Autodesk Fusion 360 part; units mm, degrees
sketch "Sketch1" plane through (0, 0, 0) normal (0, 1, 0) x (1, 0, 0)
  line L0 (-67.5, -70) -> (67.5, -70)
  line L1 (70, -67.5) -> (70, 67.5)
  line L2 (67.5, 70) -> (-67.5, 70)
  line L3 (-70, 67.5) -> (-70, -67.5)
  line L4 (-70, -70) -> (70, 70) construction
  line L5 (70, -70) -> (-70, 70) construction
  arc A0 (-67.5, 70) -> (-70, 67.5) centre (-67.5, 67.5) ccw
  arc A1 (70, 67.5) -> (67.5, 70) centre (67.5, 67.5) ccw
  arc A2 (67.5, -70) -> (70, -67.5) centre (67.5, -67.5) ccw
  arc A3 (-70, -67.5) -> (-67.5, -70) centre (-67.5, -67.5) ccw
  dimension "d1" = 140
  dimension "d2" = 140
  dimension "d25" = 2.5
  dimension "d26" = 2.5
  dimension "d27" = 2.5
  dimension "d28" = 2.5
extrude "Extrude1" add sketch "Sketch1" along normal blind 3
sketch "Sketch11" plane through (0, 0, 0) normal (0, -1, 0) x (1, 0, 0)
  arc A0 (-67.5, 70) -> (-70, 67.5) centre (-67.5, 67.5) ccw
  line L0 (-70, 67.5) -> (-70, -67.5)
  arc A1 (-70, -67.5) -> (-67.5, -70) centre (-67.5, -67.5) ccw
  line L1 (-67.5, -70) -> (67.5, -70)
  arc A2 (67.5, -70) -> (70, -67.5) centre (67.5, -67.5) ccw
  line L2 (70, -67.5) -> (70, 67.5)
  arc A3 (70, 67.5) -> (67.5, 70) centre (67.5, 67.5) ccw
  line L3 (67.5, 70) -> (-67.5, 70)
  line L4 (37.5, 38.65) -> (37.5, 51.35)
  line L5 (-37.5, 51.35) -> (-37.5, 38.65)
  line L6 (-51.35, -37.5) -> (-38.65, -37.5)
  line L7 (-38.65, 37.5) -> (-51.35, 37.5)
  line L8 (37.5, -51.35) -> (37.5, -38.65)
  line L9 (-37.5, -38.65) -> (-37.5, -51.35)
  line L10 (38.65, -37.5) -> (51.35, -37.5)
  line L11 (51.35, 37.5) -> (38.65, 37.5)
  circle A4 centre (-22, -45) radius 2.1
  circle A5 centre (-32, -45) radius 2.1
  circle A6 centre (22, -45) radius 2.1
  circle A7 centre (32, -45) radius 2.1
  circle A8 centre (-45, -22) radius 2.1
  circle A9 centre (-45, -32) radius 2.1
  circle A10 centre (-45, 22) radius 2.1
  circle A11 centre (-45, 32) radius 2.1
  circle A12 centre (-32, 45) radius 2.1
  circle A13 centre (-22, 45) radius 2.1
  circle A14 centre (22, 45) radius 2.1
  circle A15 centre (32, 45) radius 2.1
  circle A16 centre (45, 22) radius 2.1
  circle A17 centre (45, 32) radius 2.1
  circle A18 centre (45, -22) radius 2.1
  circle A19 centre (45, -32) radius 2.1
  line L12 (-51.35, 37.5) -> (-38.65, 37.5)
  line L13 (-38.65, 37.5) -> (-38.65, 16.5)
  line L14 (-38.65, 16.5) -> (-51.35, 16.5)
  line L15 (-51.35, 16.5) -> (-51.35, 37.5)
  line L16 (-51.35, -37.5) -> (-38.65, -37.5)
  line L17 (-38.65, -37.5) -> (-38.65, -16.5)
  line L18 (-38.65, -16.5) -> (-51.35, -16.5)
  line L19 (-51.35, -16.5) -> (-51.35, -37.5)
  line L20 (-37.5, -51.35) -> (-16.5, -51.35)
  line L21 (-16.5, -51.35) -> (-16.5, -38.65)
  line L22 (-16.5, -38.65) -> (-37.5, -38.65)
  line L23 (-37.5, -38.65) -> (-37.5, -51.35)
  line L24 (37.5, -38.65) -> (16.5, -38.65)
  line L25 (16.5, -38.65) -> (16.5, -51.35)
  line L26 (16.5, -51.35) -> (37.5, -51.35)
  line L27 (37.5, -51.35) -> (37.5, -38.65)
  line L28 (38.65, -37.5) -> (51.35, -37.5)
  line L29 (51.35, -37.5) -> (51.35, -16.5)
  line L30 (51.35, -16.5) -> (38.65, -16.5)
  line L31 (38.65, -16.5) -> (38.65, -37.5)
  line L32 (51.35, 37.5) -> (38.65, 37.5)
  line L33 (38.65, 37.5) -> (38.65, 16.5)
  line L34 (38.65, 16.5) -> (51.35, 16.5)
  line L35 (51.35, 16.5) -> (51.35, 37.5)
  line L36 (37.5, 38.65) -> (16.5, 38.65)
  line L37 (16.5, 38.65) -> (16.5, 51.35)
  line L38 (16.5, 51.35) -> (37.5, 51.35)
  line L39 (37.5, 51.35) -> (37.5, 38.65)
  line L40 (-37.5, 38.65) -> (-16.5, 38.65)
  line L41 (-16.5, 38.65) -> (-16.5, 51.35)
  line L42 (-16.5, 51.35) -> (-37.5, 51.35)
  line L43 (-37.5, 51.35) -> (-37.5, 38.65)
  point P0 (0, 45)
  point P1 (-45, 0)
  point P2 (45, 0)
  dimension "d68" = 12.7
  dimension "d73" = 12.7
  dimension "d77" = 4.2
  dimension "d79" = 4.2
  dimension "d81" = 4.2
  dimension "d83" = 4.2
  dimension "d85" = 4.2
  dimension "d87" = 4.2
  dimension "d89" = 4.2
  dimension "d91" = 4.2
  dimension "d93" = 4.2
  dimension "d95" = 4.2
  dimension "d97" = 4.2
  dimension "d99" = 4.2
  dimension "d101" = 4.2
  dimension "d103" = 4.2
  dimension "d105" = 4.2
  dimension "d107" = 4.2
  dimension "d111" = 21
  dimension "d112" = 12.7
  dimension "d113" = 21
  dimension "d114" = 21
  dimension "d115" = 21
  dimension "d116" = 21
  dimension "d117" = 21
  dimension "d118" = 21
  dimension "d119" = 21
  dimension "d120" = 12.7
extrude "Extrude9" add sketch "Sketch11" along normal blind 5 contours L5 L40 L41 L42 L43 | L6 L16 L17 L18 L19 | L8 L24 L25 L26 L27 | L11 L32 L33 L34 L35
sketch "Sketch14" plane through (0, 0, 0) normal (0, -1, 0) x (-1, 0, 0)
  line L0 (51.35, 16.5) -> (38.65, 16.5)
  line L1 (38.65, 16.5) -> (38.65, 37.5)
  line L2 (38.65, 37.5) -> (51.35, 37.5)
  line L3 (51.35, 37.5) -> (51.35, 16.5)
  line L4 (37.5, -51.35) -> (16.5, -51.35)
  line L5 (16.5, -51.35) -> (16.5, -38.65)
  line L6 (16.5, -38.65) -> (37.5, -38.65)
  line L7 (37.5, -38.65) -> (37.5, -51.35)
  line L8 (-37.5, 51.35) -> (-16.5, 51.35)
  line L9 (-16.5, 51.35) -> (-16.5, 38.65)
  line L10 (-16.5, 38.65) -> (-37.5, 38.65)
  line L11 (-37.5, 38.65) -> (-37.5, 51.35)
  line L12 (-51.35, -16.5) -> (-38.65, -16.5)
  line L13 (-38.65, -16.5) -> (-38.65, -37.5)
  line L14 (-38.65, -37.5) -> (-51.35, -37.5)
  line L15 (-51.35, -37.5) -> (-51.35, -16.5)
  arc A0 (67.5, -70) -> (70, -67.5) centre (67.5, -67.5) ccw
  line L16 (70, -67.5) -> (70, 67.5)
  arc A1 (70, 67.5) -> (67.5, 70) centre (67.5, 67.5) ccw
  line L17 (67.5, 70) -> (-67.5, 70)
  arc A2 (-67.5, 70) -> (-70, 67.5) centre (-67.5, 67.5) ccw
  line L18 (-70, 67.5) -> (-70, -67.5)
  arc A3 (-70, -67.5) -> (-67.5, -70) centre (-67.5, -67.5) ccw
  line L19 (-67.5, -70) -> (67.5, -70)
  circle A4 centre (32.5, -0.8187) radius 0.875
  circle A5 centre (32.5, -11.8187) radius 0.875
  circle A6 centre (-32.5, -11.8187) radius 0.875
  circle A7 centre (-32.5, -0.8187) radius 0.875
  circle A8 centre (32.5, -26.3187) radius 0.875
  circle A9 centre (32.5, 13.6813) radius 0.875
  circle A10 centre (-32.5, -26.3187) radius 0.875
  circle A11 centre (-32.5, 13.6813) radius 0.875
  dimension "d145" = 1.75
  dimension "d146" = 1.75
  dimension "d150" = 1.75
  dimension "d151" = 1.75
  dimension "d152" = 14.5
  dimension "d153" = 1.75
  dimension "d154" = 14.5
  dimension "d155" = 1.75
  dimension "d156" = 1.75
  dimension "d157" = 1.75
extrude "Extrude12" add sketch "Sketch14" along normal blind 7 contours A4 | A5 | A6 | A7 | A8 | A9 | A10 | A11
move_body "Move3" [suppressed]
sketch "Sketch16" plane through (0, 3, 0) normal (0, 1, 0) x (-1, 0, 0)
  circle A0 centre (45, -32) radius 2.1
  circle A1 centre (45, -22) radius 2.1
  circle A2 centre (-22, -45) radius 2.1
  circle A3 centre (-32, -45) radius 2.1
  circle A4 centre (-45, 22) radius 2.1
  circle A5 centre (-45, 32) radius 2.1
  circle A6 centre (32, 45) radius 2.1
  circle A7 centre (22, 45) radius 2.1
  point P0 (45, -32)
  point P1 (45, -22)
  point P2 (-22, -45)
  point P3 (-32, -45)
  point P4 (-45, 22)
  point P5 (-45, 32)
  point P6 (32, 45)
  point P7 (22, 45)
  dimension "d162" = 4.2
  dimension "d163" = 4.2
  dimension "d164" = 4.2
  dimension "d165" = 4.2
  dimension "d166" = 4.2
  dimension "d167" = 4.2
  dimension "d168" = 4.2
  dimension "d169" = 4.2
hole "Hole5" at (-45, 3, -32) at (-45, 3, -22) at (-32, 3, 45) at (-22, 3, 45) at (45, 3, 22) at (45, 3, 32) at (22, 3, -45) at (32, 3, -45) direction (0, -1, 0) diameter 4.2 depth 5 tip angle 180 counterbore diameter 7.5 counterbore depth 5
Design review of the part built by this model. Coordinates are the model's own, in mm. A direction names the side the tool comes from. Round coordinates to 2 decimals unless told otherwise and drop trailing zeros. Write each loop counter-clockwise with the first axis right and the second up, starting at its lowest first coordinate (ties: lowest second). Pieces come first, ordered by that corner, then holes. Notation, with made-up numbers: (74, 6) -> (78, 6) arc R16 ccw to (78, 35) -> close; hole circle Ø11 at (11, 82.5). An arc over 180 degrees is marked (long way). One line per question, with ' | ' between items.
(1) Take a section at C-C, the plane x = -45. State the section outline as (y, z) points.
Result sheet:
outline: (-5, -37.5) -> (0, -37.5) -> (0, -70) -> (3, -70) -> (3, -35.75) -> (-2, -35.75) -> (-2, -34.1) -> (-5, -34.1) -> close; (-5, -29.9) -> (-2, -29.9) -> (-2, -28.25) -> (3, -28.25) -> (3, -25.75) -> (-2, -25.75) -> (-2, -24.1) -> (-5, -24.1) -> close; (-5, -19.9) -> (-2, -19.9) -> (-2, -18.25) -> (3, -18.25) -> (3, 70) -> (0, 70) -> (0, -16.5) -> (-5, -16.5) -> close
(2) Insertion check: P1, Ø1.5, axis at x = 44.5, y = -2, coming from the -Z side; P2, Ø1.5, axis at x = -43, y = -3, coming from the +Z side; P3, Ø2.5, axis at x = -30, y = -1.5, coming from the +Z side. Each pin has a flat end and moves straight along its axis. Give the tip position at first contact, or say it passes through.
Result sheet:
P1: z = 16.5 | P2: z = -16.5 | P3: z = 51.35
(3) Machinability: for faces 1 (the flat face through (70, 1, 1)), 2 (the flat face through (47, -2, 24)), 3 (the cylindrical face through (46.13, -3.48, 20.23)), 4 (the flat face through (45, -2, 37.5)), 5 (the flat face through (-1, 0, -1)), which of the approach directions +Z, -Z, +X, -X, +Y, -Y give a long, thin tool a straight path to every point of the face, cutting with its end or side? Answer none if there is none.
Result sheet:
face 1: +Z, -Z, +X, +Y, -Y | face 2: +Y | face 3: +Y, -Y | face 4: +Z, +X, -X, -Y | face 5: -Y
(4) Take a section at B-B, the plane z = 32. State the section outline as (x, y) points, and give its area (3 significant figures).
Result sheet:
outline: (-70, 0) -> (38.65, 0) -> (38.65, -5) -> (42.9, -5) -> (42.9, -2) -> (41.25, -2) -> (41.25, 3) -> (-70, 3) -> close; (47.1, -5) -> (51.35, -5) -> (51.35, 0) -> (70, 0) -> (70, 3) -> (48.75, 3) -> (48.75, -2) -> (47.1, -2) -> close | area: 433 mm2
(5) Take a section at A-A, the plane x = -22. State the section outline as (y, z) points, and give its area (3 significant figures).
Result sheet:
outline: (-5, 38.65) -> (0, 38.65) -> (0, -70) -> (3, -70) -> (3, 41.25) -> (-2, 41.25) -> (-2, 42.9) -> (-5, 42.9) -> close; (-5, 47.1) -> (-2, 47.1) -> (-2, 48.75) -> (3, 48.75) -> (3, 70) -> (0, 70) -> (0, 51.35) -> (-5, 51.35) -> close | area: 433 mm2
(6) Draft analysis for pull direction X (two halves, no side actions). For faces 6 (the flat face through (27, -5, -45)), 7 (the flat face through (16.5, -2, -45)), 8 (the cylindrical face through (-43.87, -3.48, -23.77)), state which applies: released by +X, released by -X, zero draft, split by the parting line, or undercut.
Result sheet:
face 6: zero draft | face 7: released by -X | face 8: undercut
(7) Wall thickness on line 1 (Z direction, x = -45, y = -3.25); line 2 (X direction, y = 1.7, z = -45); line 3 (X direction, y = -0.05, z = -45): over which ranges is each line inside the solid? List them lowest first. Write a range as [from, to].
Result sheet:
line 1: [-37.5, -34.1], [-29.9, -24.1], [-19.9, -16.5] | line 2: [-70, 18.25], [25.75, 28.25], [35.75, 70] | line 3: [16.5, 18.25], [25.75, 28.25], [35.75, 37.5]
